Verification items for the finished model (mm, model axes). Coordinates: 2 decimals unless noted, no trailing zeros. Order: outer loops, then holes, each group sorted by start corner. A loop starts at its lowest first (then second) coordinate and runs counter-clockwise, first axis right, second up. Notation, with made-up numbers: (0.5, 85) - (45.5, 85) arc R22 ccw to (45.5, 91) - close; hole circle Ø5 at (19, 53). An arc over 180 degrees is marked (long way). Answer as CSV lines item,"result". Start each with the question number.
1. Section check B-B (x = -43.5). Record the cut outline in (y, z), and give its area (3 significant figures).
2. Go/stop test with flat-tipped pins: pin 1 (1.5 mm diameter, centred on x = -20, y = -3.5, fed in from +Z); pin 2 (2 mm diameter, centred on x = 2, y = -3.5, fed in from +Z). Record where each tip stops, or that it passes through.
3. Section check A-A (y = -7). Record the cut outline in (x, z), and give its area (3 significant figures).
4. Material ranges on L1, parallel to X at y = -5.5, z = 92.5; L2, parallel to X at y = -6.5, z = -47.5; L3, parallel to Z at x = 22.5, y = -5.5, recorded low to high. Write a range as [from, to].
5. Section check C-C (z = -28). Record the cut outline in (x, y).
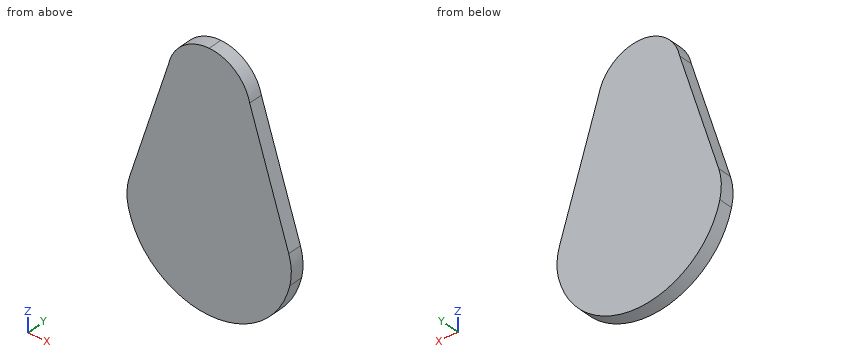
from build123d import *

# Parameters (mm, degrees)
F1_DEPTH = 10


with BuildPart() as f1:
    # F0 (on Front) → F1 (new body)
    with BuildSketch(Plane.XZ):
        with BuildLine():
            ThreePointArc((-57.586286, 7.57811), (-59.44227, -2.996741), (-58.418656, -13.684322))
            ThreePointArc((-58.418656, -13.684322), (0, -60), (58.418656, -13.684322))
            ThreePointArc((58.418656, -13.684322), (59.44227, -2.996741), (57.586286, 7.57811))
            Line((57.586286, 7.57811), (29.338606, 96.264676))
            ThreePointArc((29.338606, 96.264676), (18.868753, 113.323168), (0, 120))
            ThreePointArc((0, 120), (-18.868753, 113.323168), (-29.338606, 96.264676))
            Line((-29.338606, 96.264676), (-57.586286, 7.57811))
        make_face()
    extrude(amount=F1_DEPTH)


solid = f1.part
Evaluation:
1,outline,"(-10, -41.32) - (0, -41.32) - (0, 51.8) - (-10, 51.8) - close"
1,area,"931 mm²"
2,pin 1,"stops at z = 113.01"
2,pin 2,"stops at z = 119.98"
3,outline,"(-58.42, -13.68) arc R60 ccw to (58.42, -13.68) arc R40 ccw to (57.59, 7.58) - (29.34, 96.26) arc R30 ccw to (0, 120) arc R30 ccw to (-29.34, 96.26) - (-57.59, 7.58) arc R40 ccw to start"
3,area,"15,300 mm²"
4,L1,"x = [-30.54, 30.54]"
4,L2,"x = [-36.66, 36.66]"
4,L3,"z = [-55.62, 109.84]"
5,outline,"(-53.07, -10) - (53.07, -10) - (53.07, 0) - (-53.07, 0) - close"
